Job drawing, mm, ordinate dimensions from the low corner. One solid piece. A direction names the side the tool comes from. Coordinates: 2 decimals unless noted, no trailing zeros. Write each loop counter-clockwise with the first axis right and the second up, starting at its lowest first coordinate (ties: lowest second). Pieces come first, ordered by that corner, then holes.
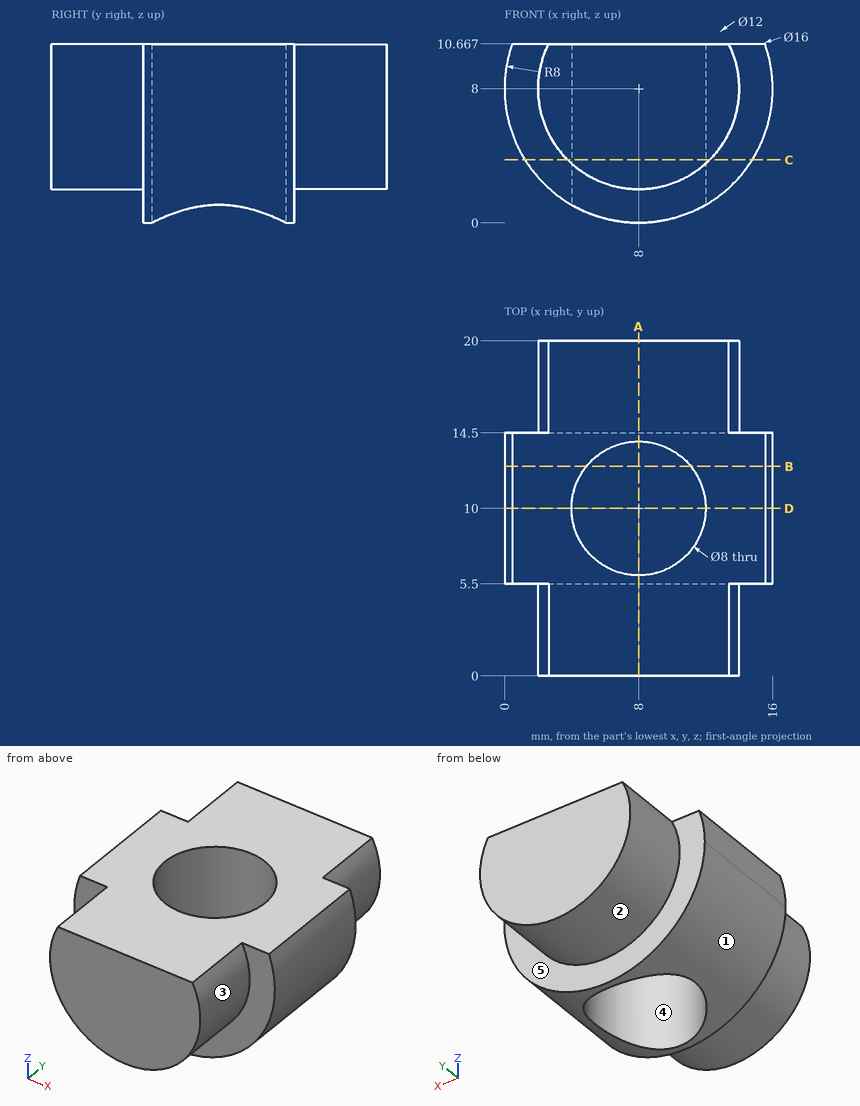
1. Saw through at C-C on z = 3.75. List the corners of the cut face in (x, y) (1 decimal).
Computed values:
outline: (1.2, 5.5) - (3.8, 5.5) - (3.8, 0) - (12.2, 0) - (12.2, 5.5) - (14.8, 5.5) - (14.8, 14.5) - (12.2, 14.5) - (12.2, 20) - (3.8, 20) - (3.8, 14.5) - (1.2, 14.5) - close; hole circle Ø8 at (8, 10)
2. Flat gauge pins, fed straight in: pin 1 (1 mm diameter, centred on y = 7.5, z = 9.5, fed in from +X); pin 2 (3 mm diameter, centred on y = 13.5, z = 4.5, fed in from -X); pin 3 (1 mm diameter, centred on x = 2.5, y = 9.5, fed in from -Z) (1 decimal). Where does each tip first touch, or does it go through?
Computed values:
pin 1: stops at x = 15.94
pin 2: stops at x = 0.25
pin 3: stops at z = 1.8
3. Saw through at A-A on x = 8. List the corners of the cut face in (y, z), plus the area to 3 significant figures.
Computed values:
outline: (0, 2) - (5.5, 2) - (5.5, 0) - (6, 0) - (6, 10.67) - (0, 10.67) - close; (14, 0) - (14.5, 0) - (14.5, 2) - (20, 2) - (20, 10.67) - (14, 10.67) - close
area: 106 mm2
4. Mould opens along Y. For the marked faces 3, 4 and 5 say: +Y half, -Y half, draft (parallel to the pull), parting line (faces both ways), or undercut.
Computed values:
face 3: draft
face 4: undercut
face 5: +Y half
5. Saw through at D-D on y = 10. List the corners of the cut face in (x, z).
Computed values:
outline: (0, 8) arc R8 ccw to (4, 1.07) - (4, 10.67) - (0.46, 10.67) arc R8 ccw to start; (12, 1.07) arc R8 ccw to (15.54, 10.67) - (12, 10.67) - close
6. Saw through at B-B on y = 12.5. List the corners of the cut face in (x, z) (1 decimal).
Computed values:
outline: (0, 8) arc R8 ccw to (4.9, 0.6) - (4.9, 10.7) - (0.5, 10.7) arc R8 ccw to start; (11.1, 0.6) arc R8 ccw to (15.5, 10.7) - (11.1, 10.7) - close
7. Probe line 1 along Y through (x, z) = (8, 8); line 2 along Y through (x, z) = (3.25, 2.25); line 3 along X through (y, z) = (3, 8). List the from-to ranges inside material, lowest first.
Computed values:
line 1: y = 0 to 6, 14 to 20
line 2: y = 5.5 to 14.5
line 3: x = 2 to 14
8. 3-axis set-ups, long thin cutter, end or side, ignore diameter. For the marked faces 1 and 2: which of +Z, -Z, +X, -X, +Y, -Y reach the whole face in a straight line?
Computed values:
face 1: +Y, -Y
face 2: +Y
